from build123d import *

# Parameters (mm, degrees)
SKETCH1_W               = 42
SKETCH1_H               = 42
BOSS_EXTRUDE1_DEPTH     = 33.95
SKETCH2_R               = 11
BOSS_EXTRUDE2_DEPTH     = 0.85
SKETCH3_R               = 2.5
BOSS_EXTRUDE3_DEPTH     = 22
CUT_EXTRUDE_THIN1_DEPTH = 75.110795435
M3_TAPPED_HOLE1_D       = 2.5
M3_TAPPED_HOLE1_DEPTH   = 4.248924226
M3_TAPPED_HOLE1_TIP     = 0.751075774


with BuildPart() as part:
    # Sketch1 → Boss-Extrude1 (new, symmetric)
    with BuildSketch(Plane.XY):
        Rectangle(SKETCH1_W, SKETCH1_H)
    extrude(amount=BOSS_EXTRUDE1_DEPTH, both=True)

    # Sketch2 → Boss-Extrude2 (add, symmetric)
    with BuildSketch(Plane.XY.offset(33.95)):
        with Locations(Location((0, 0, 0), (0, 0, 180))):
            Circle(SKETCH2_R)
    extrude(amount=BOSS_EXTRUDE2_DEPTH, both=True)

    # Sketch3 → Boss-Extrude3 (add)
    with BuildSketch(Plane.XY.offset(34.8)):
        Circle(SKETCH3_R)
    extrude(amount=BOSS_EXTRUDE3_DEPTH)

    # Sketch4 → Cut-Extrude-Thin1 (cut, through all)
    with BuildSketch(Plane.XY.offset(33.95)):
        Polygon((0, 52.113769773), (52.113769773, 0), (0, -52.113769773), (-52.113769773, 0), align=None)
        Polygon((0, 37.97163415), (37.97163415, 0), (0, -37.97163415), (-37.97163415, 0), align=None, mode=Mode.SUBTRACT)
    extrude(amount=-CUT_EXTRUDE_THIN1_DEPTH, mode=Mode.SUBTRACT)

    # M3 Tapped Hole1
    with Locations(Plane.XY.offset(33.95)):
        with Locations((-15.5, 15.5), (15.5, -15.5), (15.5, 15.5), (-15.5, -15.5)):
            Hole(M3_TAPPED_HOLE1_D / 2, depth=M3_TAPPED_HOLE1_DEPTH)
            with Locations((0, 0, -(M3_TAPPED_HOLE1_DEPTH + M3_TAPPED_HOLE1_TIP / 2))):  # 118° drill point
                Cone(0, M3_TAPPED_HOLE1_D / 2, M3_TAPPED_HOLE1_TIP, mode=Mode.SUBTRACT)


solid = part.part
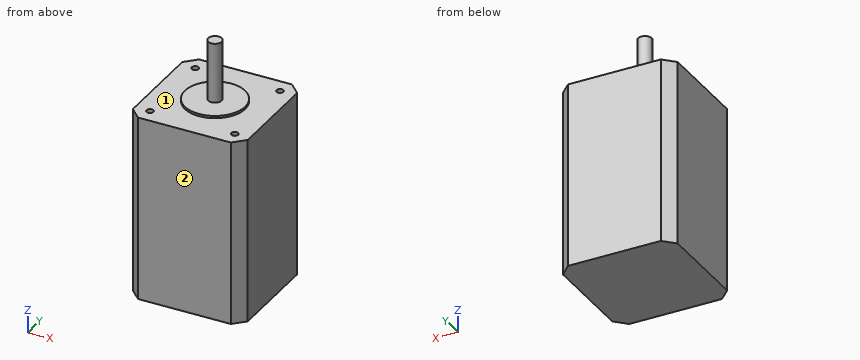
Build history of the part. All positions in model axes, mm. Face numbers are marked on the shaded views. A direction names the side the tool comes from. Round coordinates to 2 decimals unless told otherwise and drop trailing zeros. Loops run counter-clockwise (first coordinate to the right, second up) from the corner with the lowest first, then second, coordinate; pieces in that order, holes last. Notation, with made-up numbers: (57, 15.25) -> (89, 15.25) arc R15 cw to (89, 42.25) -> close; hole circle Ø7 at (67, 14.5). An arc over 180 degrees is marked (long way). One line per item, written item: value. Start each with the question number.
Q1. Drop flat-ended pins along their axis: pin 1 Ø12.5 at (x, y) = (1.5, 2.5) entering from +Z; pin 2 Ø1.5 at (x, y) = (-15.5, -15.5) entering from +Z; pin 3 Ø8 at (x, z) = (12.5, 42) entering from +Y. Give the stop position or say it passes through.
Q2. Probe line 1 along Y through (x, z) = (15.5, 32.3); line 2 along X through (y, z) = (-15, 32). List the from-to ranges inside material, lowest first.
Q3. Cut at B-B on x = 0. List the corners of the cut face in (y, z), plus the area to 3 significant figures.
Q4. 3-axis set-ups, long thin cutter, end or side, ignore diameter. For the marked faces 1 and 2: which of +Z, -Z, +X, -X, +Y, -Y reach the whole face in a straight line?
Q5. Cut at A-A on z = 32. List the corners of the cut face in (x, y).
Q6. Cut at D-D on z = -26. List the corners of the cut face in (x, y).
Computed:
1. pin 1: z = 56.8
1. pin 2: z = 29.4
1. pin 3: through
2. line 1: -21 to -16.75, -14.25 to 14.25, 16.75 to 21
2. line 2: -21 to -16.65, -14.35 to 14.35, 16.65 to 21
3. outline: (-21, -33.95) -> (21, -33.95) -> (21, 33.95) -> (11, 33.95) -> (11, 34.8) -> (2.5, 34.8) -> (2.5, 56.8) -> (-2.5, 56.8) -> (-2.5, 34.8) -> (-11, 34.8) -> (-11, 33.95) -> (-21, 33.95) -> close
3. area: 2,980 mm²
4. face 1: +Z
4. face 2: +Z, -Z, +X, -X, -Y
5. outline: (-21, -16.97) -> (-16.97, -21) -> (16.97, -21) -> (21, -16.97) -> (21, 16.97) -> (16.97, 21) -> (-16.97, 21) -> (-21, 16.97) -> close; hole circle Ø2.5 at (-15.5, -15.5); hole circle Ø2.5 at (-15.5, 15.5); hole circle Ø2.5 at (15.5, -15.5); hole circle Ø2.5 at (15.5, 15.5)
6. outline: (-21, -16.97) -> (-16.97, -21) -> (16.97, -21) -> (21, -16.97) -> (21, 16.97) -> (16.97, 21) -> (-16.97, 21) -> (-21, 16.97) -> close
